The model under review builds one solid part; all positions refer to its coordinate system, in mm. A direction names the side the tool comes from. Round coordinates to 2 decimals unless told otherwise and drop trailing zeros. Write each loop counter-clockwise with the first axis right and the second up, starting at its lowest first coordinate (ties: lowest second). Pieces come first, ordered by that corner, then holes. Notation, with made-up numbers: (-37.5, 32) -> (-11.5, 32) arc R30 cw to (-11.5, 59) -> close; hole circle Ø10 at (-19, -25). An arc over 180 degrees is marked (long way). Use CSV: the item, a comma, the result in double quotes. Start each with the question number.
1) Machinability: for faces 3 (the face through (-27.606, 39.26, 5.08)), 4 (the face through (-12, 20, 0)), 5 (the face through (-20, 28, 25)), 6 (the face through (-34, 20, 25)), which of the approach directions +Z, -Z, +X, -X, +Y, -Y give a long, thin tool a straight path to every point of the face, cutting with its end or side? Answer none if there is none.
2) Wall thickness on probe 1 along Z at (x, y) = (-36.25, 20); probe 2 along Y at (x, z) = (-10, 6); probe 3 along Y at (x, z) = (-9.65, 35): over which ranges is each line inside the solid? List them lowest first. Write a range as [from, to].
3) Take a section at B-B, the plane z = 35. Give the boundary of the cut face in (x, y), then the cut area to 4 significant figures.
4) Take a section at A-A, the plane y = 36. Give the boundary of the cut face in (x, z), then the cut area to 3 significant figures.
5) For pin 1 Ø1 at (y, z) = (28.5, -1) entering from -X; pin 2 Ø6.5 at (y, z) = (16, 35) entering from +X, all flat-tipped, find the tip position at first contact; note any pin that passes through.
6) Take a section at C-C, the plane x = -10. State how many separate pieces and enclosed holes the cut face has, then the cut area to 3 significant figures.
7) Mouldability with a two-part tool opening along Y and no side actions: class faces 1 (the face through (-20, 20, -7)), 2 (the face through (-34, 26.25, -1)) as released by +Y, released by -Y, zero draft, split by the parting line, or undercut.
from build123d import *

# Parameters (mm, degrees)
ESQUISSE1_W              = 40
ESQUISSE1_H              = 40
BOSS_EXTRU_1_DEPTH       = 50
ESQUISSE2_R              = 5
ENL_V_MAT_EXTRU_1_DEPTH  = 41
ESQUISSE3_R              = 5
ENL_V_MAT_EXTRU_2_DEPTH  = 41
ESQUISSE4_W              = 20
ESQUISSE4_H              = 14
ENL_V_MAT_EXTRU_3_DEPTH  = 29
ESQUISSE5_W              = 14
ESQUISSE5_H              = 20
ENL_V_MAT_EXTRU_4_DEPTH  = 29
ESQUISSE6_W              = 22
ESQUISSE6_H              = 14
ENL_V_MAT_EXTRU_5_DEPTH  = 24
ESQUISSE7_W              = 14
ESQUISSE7_H              = 22
ENL_V_MAT_EXTRU_6_DEPTH  = 24
ESQUISSE8_R              = 11
ENL_V_MAT_EXTRU_7_DEPTH  = 7
ESQUISSE9_R              = 12.5
ENL_V_MAT_EXTRU_8_DEPTH  = 1.5
ESQUISSE10_R             = 11
ENL_V_MAT_EXTRU_9_DEPTH  = 7
ESQUISSE11_R             = 12.5
ENL_V_MAT_EXTRU_10_DEPTH = 1.5
ESQUISSE12_W             = 40
ESQUISSE12_H             = 40
BOSS_EXTRU_2_DEPTH       = 7
ESQUISSE13_R             = 2.25
ENL_V_MAT_EXTRU_11_DEPTH = 15
ESQUISSE14_W             = 3.5
ESQUISSE14_H             = 7.5
ENL_V_MAT_EXTRU_12_DEPTH = 12
ESQUISSE15_W             = 7.5
ESQUISSE15_H             = 3.5
ENL_V_MAT_EXTRU_13_DEPTH = 12


with BuildPart() as part:
    # Esquisse1 → Boss.-Extru.1 (new body)
    with BuildSketch(Plane.XY):
        with Locations((-20, 20)):
            Rectangle(ESQUISSE1_W, ESQUISSE1_H)
    extrude(amount=BOSS_EXTRU_1_DEPTH)

    # Esquisse2 → Enlèv. mat.-Extru.1 (cut, through all)
    with BuildSketch(Plane(origin=(0, 40, 0), x_dir=(1, 0, 0), z_dir=(0, 1, 0))):
        with Locations(Location((-20, -15, 0), (0, 0, 270))):  # turned: the seam where the file's is
            Circle(ESQUISSE2_R)
    extrude(amount=-ENL_V_MAT_EXTRU_1_DEPTH, mode=Mode.SUBTRACT)

    # Esquisse3 → Enlèv. mat.-Extru.2 (cut, through all)
    with BuildSketch(Plane.ZY.offset(40)):
        with Locations((35, 20)):
            Circle(ESQUISSE3_R)
    extrude(amount=-ENL_V_MAT_EXTRU_2_DEPTH, mode=Mode.SUBTRACT)

    # Esquisse4 → Enlèv. mat.-Extru.3 (cut)
    with BuildSketch(Plane.ZY.offset(40)):
        with Locations((15, 20)):
            Rectangle(ESQUISSE4_W, ESQUISSE4_H)
    extrude(amount=-ENL_V_MAT_EXTRU_3_DEPTH, mode=Mode.SUBTRACT)

    # Esquisse5 → Enlèv. mat.-Extru.4 (cut)
    with BuildSketch(Plane.XZ):
        with Locations((-20, 35)):
            Rectangle(ESQUISSE5_W, ESQUISSE5_H)
    extrude(amount=-ENL_V_MAT_EXTRU_4_DEPTH, mode=Mode.SUBTRACT)

    # Esquisse6 → Enlèv. mat.-Extru.5 (cut)
    with BuildSketch(Plane(origin=(0, 0, 0), x_dir=(0, 0, -1), z_dir=(1, 0, 0))):
        with Locations((-11, 20)):
            Rectangle(ESQUISSE6_W, ESQUISSE6_H)
    extrude(amount=-ENL_V_MAT_EXTRU_5_DEPTH, mode=Mode.SUBTRACT)

    # Esquisse7 → Enlèv. mat.-Extru.6 (cut)
    with BuildSketch(Plane(origin=(0, 40, 0), x_dir=(1, 0, 0), z_dir=(0, 1, 0))):
        with Locations((-20, -39)):
            Rectangle(ESQUISSE7_W, ESQUISSE7_H)
    extrude(amount=-ENL_V_MAT_EXTRU_6_DEPTH, mode=Mode.SUBTRACT)

    # Esquisse8 → Enlèv. mat.-Extru.7 (cut)
    with BuildSketch(Plane(origin=(0, 0, 0), x_dir=(0, 0, -1), z_dir=(1, 0, 0))):
        with Locations(Location((-35, 20, 0), (0, 0, 90))):  # turned: the seam where the file's is
            Circle(ESQUISSE8_R)
    extrude(amount=-ENL_V_MAT_EXTRU_7_DEPTH, mode=Mode.SUBTRACT)

    # Esquisse9 → Enlèv. mat.-Extru.8 (cut)
    with BuildSketch(Plane(origin=(0, 0, 0), x_dir=(0, 0, -1), z_dir=(1, 0, 0))):
        with Locations(Location((-35, 20, 0), (0, 0, 90))):  # turned: the seam where the file's is
            Circle(ESQUISSE9_R)
    extrude(amount=-ENL_V_MAT_EXTRU_8_DEPTH, mode=Mode.SUBTRACT)

    # Esquisse10 → Enlèv. mat.-Extru.9 (cut)
    with BuildSketch(Plane(origin=(0, 40, 0), x_dir=(1, 0, 0), z_dir=(0, 1, 0))):
        with Locations(Location((-20, -15, 0), (0, 0, 270))):  # turned: the seam where the file's is
            Circle(ESQUISSE10_R)
    extrude(amount=-ENL_V_MAT_EXTRU_9_DEPTH, mode=Mode.SUBTRACT)

    # Esquisse11 → Enlèv. mat.-Extru.10 (cut)
    with BuildSketch(Plane(origin=(0, 40, 0), x_dir=(1, 0, 0), z_dir=(0, 1, 0))):
        with Locations(Location((-20, -15, 0), (0, 0, 270))):  # turned: the seam where the file's is
            Circle(ESQUISSE11_R)
    extrude(amount=-ENL_V_MAT_EXTRU_10_DEPTH, mode=Mode.SUBTRACT)

    # Esquisse12 → Boss.-Extru.2 (add)
    with BuildSketch(Plane(origin=(0, 0, 0), x_dir=(-1, 0, 0), z_dir=(0, 0, -1))):
        with Locations((20, 20)):
            Rectangle(ESQUISSE12_W, ESQUISSE12_H)
    extrude(amount=BOSS_EXTRU_2_DEPTH)

    # Esquisse13 → Enlèv. mat.-Extru.11 (cut)
    with BuildSketch(Plane(origin=(0, 0, -7), x_dir=(-1, 0, 0), z_dir=(0, 0, -1))):
        with Locations((10, 7.5)):
            Circle(ESQUISSE13_R)
        with Locations((32.5, 30)):
            Circle(ESQUISSE13_R)
    extrude(amount=-ENL_V_MAT_EXTRU_11_DEPTH, mode=Mode.SUBTRACT)

    # Esquisse14 → Enlèv. mat.-Extru.12 (cut)
    with BuildSketch(Plane.ZY.offset(40)):
        with Locations((-1.25, 30)):
            Rectangle(ESQUISSE14_W, ESQUISSE14_H)
    extrude(amount=-ENL_V_MAT_EXTRU_12_DEPTH, mode=Mode.SUBTRACT)

    # Esquisse15 → Enlèv. mat.-Extru.13 (cut)
    with BuildSketch(Plane.XZ):
        with Locations((-10, -1.25)):
            Rectangle(ESQUISSE15_W, ESQUISSE15_H)
    extrude(amount=-ENL_V_MAT_EXTRU_13_DEPTH, mode=Mode.SUBTRACT)


solid = part.part
Values found:
1,face 3,"+Y"
1,face 4,"+X"
1,face 5,"+Z, -Y"
1,face 6,"-X"
2,probe 1,"[-7, 5], [25, 30], [40, 50]"
2,probe 2,"[0, 5.25], [9.75, 13], [27, 40]"
2,probe 3,"[0, 15], [25, 40]"
3,outline,"(-40, 0) -> (-27, 0) -> (-27, 15) -> (-40, 15) -> close; (-40, 25) -> (-27, 25) -> (-27, 40) -> (-40, 40) -> close; (-13, 0) -> (0, 0) -> (0, 7.5) -> (-1.5, 7.5) -> (-1.5, 9) -> (-7, 9) -> (-7, 15) -> (-13, 15) -> close; (-13, 25) -> (-7, 25) -> (-7, 31) -> (-1.5, 31) -> (-1.5, 32.5) -> (0, 32.5) -> (0, 40) -> (-13, 40) -> close"
3,area,"691.5 mm²"
4,outline,"(-40, -7) -> (0, -7) -> (0, 50) -> (-13, 50) -> (-13, 28) -> (-27, 28) -> (-27, 50) -> (-40, 50) -> close; hole circle Ø22 at (-20, 15)"
4,area,"1,590 mm²"
5,pin 1,"x = -28"
5,pin 2,"x = -7"
6,separate pieces,"2"
6,enclosed holes,"2"
6,area,"1,730 mm²"
7,face 1,"zero draft"
7,face 2,"undercut"
